```python
from build123d import *

# Parameters (mm, degrees)
SKETCH1_R           = 1.4225
SKETCH1_R_2         = 1.450000001
SKETCH1_R_3         = 3.250000001
SKETCH1_R_4         = 1.45
BOSS_EXTRUDE2_DEPTH = 9
FILLET1_R           = 3
FILLET2_R           = 3


with BuildPart() as part:
    # Sketch1 → Boss-Extrude2 (new body)
    with BuildSketch(Plane.XY):
        with BuildLine():
            Line((-134.22032992, 11.211856555), (-30.257718346, 11.989277985))
            ThreePointArc((-30.257718346, 11.989277985), (-25.422812351, 8.063130211), (-23.849365383, 2.036919381))
            ThreePointArc((-23.849365383, 2.036919381), (-21.809168303, -5.524545992), (-18.937059892, -12.810776569))
            Line((-18.937059892, -12.810776569), (43.522166186, 18.694700379))
            ThreePointArc((43.522166186, 18.694700379), (46.880190718, 17.588503631), (45.77399397, 14.230479099))
            Line((45.77399397, 14.230479099), (-16.685232108, -17.274997849))
            ThreePointArc((-16.685232108, -17.274997849), (60.631470485, -51.68820799), (114.585866087, 13.511981637))
            ThreePointArc((114.585866087, 13.511981637), (55.491058325, 85.617703959), (-22.83660712, 35.058745089))
            ThreePointArc((-22.83660712, 35.058745089), (-25.272857454, 27.800559204), (-30.257718346, 21.989557576))
            Line((-30.257718346, 21.989557576), (-134.295106773, 21.211576972))
            ThreePointArc((-134.295106773, 21.211576972), (-139.257578555, 16.174328337), (-134.22032992, 11.211856555))
        make_face()
        with Locations((44.661222783, 22.812576138)):
            Circle(SKETCH1_R, mode=Mode.SUBTRACT)
        with Locations((-17.105082345, -0.346542621)):
            Circle(SKETCH1_R_2, mode=Mode.SUBTRACT)
        with Locations((-134.257718346, 16.211716764)):
            Circle(SKETCH1_R_3, mode=Mode.SUBTRACT)
        with Locations((-17.234763001, 32.78783805)):
            Circle(SKETCH1_R_2, mode=Mode.SUBTRACT)
        with Locations((-10.886578119, 48.272992738)):
            Circle(SKETCH1_R_2, mode=Mode.SUBTRACT)
        with Locations((-19.351394551, 16.203268944)):
            Circle(SKETCH1_R_2, mode=Mode.SUBTRACT)
        with Locations((-44.257717657, 16.208005084)):
            Circle(SKETCH1_R_4, mode=Mode.SUBTRACT)
        with Locations((-34.257718346, 16.211716764)):
            Circle(SKETCH1_R_4, mode=Mode.SUBTRACT)
        with Locations((-26.257718346, 16.211716764)):
            Circle(SKETCH1_R_4, mode=Mode.SUBTRACT)
        with Locations((50.992814526, 16.20404615)):
            Circle(SKETCH1_R, mode=Mode.SUBTRACT)
        with Locations((44.66019165, 10.112601289)):
            Circle(SKETCH1_R, mode=Mode.SUBTRACT)
        with Locations((106.402979176, -0.340161148)):
            Circle(SKETCH1_R_2, mode=Mode.SUBTRACT)
        with Locations((99.964508374, -15.725805073)):
            Circle(SKETCH1_R_2, mode=Mode.SUBTRACT)
        with Locations((89.779783974, -28.915040251)):
            Circle(SKETCH1_R_2, mode=Mode.SUBTRACT)
        with Locations((76.545581676, -39.022087351)):
            Circle(SKETCH1_R_2, mode=Mode.SUBTRACT)
        with Locations((61.159646121, -45.37080081)):
            Circle(SKETCH1_R_2, mode=Mode.SUBTRACT)
        with Locations((44.660635327, -47.53740903)):
            Circle(SKETCH1_R_2, mode=Mode.SUBTRACT)
        with Locations((28.159958748, -45.377056565)):
            Circle(SKETCH1_R_2, mode=Mode.SUBTRACT)
        with Locations((12.769465369, -39.03294093)):
            Circle(SKETCH1_R_2, mode=Mode.SUBTRACT)
        with Locations((-0.470981954, -28.927610099)):
            Circle(SKETCH1_R_2, mode=Mode.SUBTRACT)
        with Locations((-0.73028884, 61.593550668)):
            Circle(SKETCH1_R_2, mode=Mode.SUBTRACT)
        with Locations((12.544950118, 71.828545405)):
            Circle(SKETCH1_R_2, mode=Mode.SUBTRACT)
        with Locations((27.96860152, 78.250897654)):
            Circle(SKETCH1_R_2, mode=Mode.SUBTRACT)
        with Locations((44.528931823, 80.46247883)):
            Circle(SKETCH1_R_2, mode=Mode.SUBTRACT)
        with Locations((61.289362626, 78.261195833)):
            Circle(SKETCH1_R_2, mode=Mode.SUBTRACT)
        with Locations((76.770141151, 71.817564153)):
            Circle(SKETCH1_R_2, mode=Mode.SUBTRACT)
        with Locations((90.039018635, 61.580908601)):
            Circle(SKETCH1_R_2, mode=Mode.SUBTRACT)
        with Locations((100.202860624, 48.237837315)):
            Circle(SKETCH1_R_2, mode=Mode.SUBTRACT)
        with Locations((106.533916616, 32.776486758)):
            Circle(SKETCH1_R_2, mode=Mode.SUBTRACT)
        with Locations((108.64755512, 16.203371079)):
            Circle(SKETCH1_R_2, mode=Mode.SUBTRACT)
    extrude(amount=BOSS_EXTRUDE2_DEPTH)

    # Fillet1
    fillet1_edges = [part.edges().sort_by_distance(p)[0] for p in [
        (-18.937059892, -12.810776569, 4.5),
    ]]
    fillet(fillet1_edges, radius=FILLET1_R)

    # Fillet2
    fillet2_edges = [part.edges().sort_by_distance(p)[0] for p in [
        (-16.685232108, -17.274997849, 4.5),
    ]]
    fillet(fillet2_edges, radius=FILLET2_R)


solid = part.part
```
Verification items for the finished model (mm, model axes). A direction names the side the tool comes from. Give positions to 0.01 mm unless a question says otherwise; leave off trailing zeros. Loops run counter-clockwise (first coordinate to the right, second up) from the corner with the lowest first, then second, coordinate; pieces in that order, holes last.
1. Section check D-D, the plane x = -113. Enter the section's corners in (y, z), then the cut area to 3 significant figures.
2. Section check B-B, the plane z = 5. Count the separate pieces of the cut face and the enclosed holes in it, then the cut area to 3 significant figures.
3. Set-up check for faces 1 (the flat face through (14, 17, 9)), 2 (the flat face through (16.382, -0.595, 4.437)): record each of +Z, -Z, +X, -X, +Y, -Y from which the full face is reachable in a straight line by a thin tool's end or side.
4. Mould release check, pull along X, two halves, no side actions. Record for faces 3 (the flat face through (13.3, 3.45, 4.44)), 4 (the flat face through (14, 17, 0)), 5 (the cylindrical face through (-22.327, -3.892, 4.437)): released by +X, released by -X, zero draft, split by the parting line, or undercut.
5. Go/stop test with flat-tipped pins: pin 1 Ø2.5 at (x, y) = (27.97, 78.25) entering from +Z; pin 2 Ø4 at (x, z) = (5, 1.5) entering from -Y; pin 3 Ø1.5 at (y, z) = (-20, 7) entering from -X; pin 4 Ø1 at (x, z) = (-30.5, 5.5) entering from -Y. Record where each tip stops, or that it passes through.
6. Thickness scan on line 1 (X direction, y = -44.5, z = 8.75); line 2 (X direction, y = 77.5, z = 5.75); line 3 (X direction, y = 79.5, z = 2.5). Record the ranges inside material, lowest first.
7. Section check A-A, the plane x = 33.5. Enter the section's corners in (y, z), then the cut area to 3 significant figures.
8. Section check C-C, the plane y = 57. Enter the section's corners in (x, z), then the cut area to 3 significant figures.
Geometry says:
1. outline: (11.37, 0) - (21.37, 0) - (21.37, 9) - (11.37, 9) - close
1. area: 90.0 mm2
2. separate pieces: 1
2. enclosed holes: 30
2. area: 16,000 mm2
3. face 1: +Z, +X, -X, +Y, -Y
3. face 2: +Z, -Z
4. face 3: undercut
4. face 4: zero draft
4. face 5: released by -X
5. pin 1: passes through
5. pin 2: stops at y = -42.55
5. pin 3: stops at x = -15.4
5. pin 4: stops at y = 11.89
6. line 1: x = 10.25 to 27.01, 29.31 to 60, 62.32 to 79.05
6. line 2: x = 10.38 to 26.73, 29.21 to 60.06, 62.52 to 78.92
6. line 3: x = 14.21 to 27.23, 28.7 to 43.44, 45.61 to 60.54, 62.04 to 75.08
7. outline: (-52.64, 0) - (8.04, 0) - (8.04, 9) - (-52.64, 9) - close; (13.64, 0) - (85.57, 0) - (85.57, 9) - (13.64, 9) - close
7. area: 1,190 mm2
8. outline: (-12.42, 0) - (101.72, 0) - (101.72, 9) - (-12.42, 9) - close
8. area: 1,030 mm2
